Check sheet for the modelled part. Datum: model origin and axes. Units: mm. A direction names the side the tool comes from. Coordinates: 2 decimals unless noted, no trailing zeros. Loops run counter-clockwise (first coordinate to the right, second up) from the corner with the lowest first, then second, coordinate; pieces in that order, holes last. Notation, with made-up numbers: M 53,36.5 L 82,36.5 A10 cw 82,45.5 Z; hole C 73,18 d11. An arc over 180 degrees is marked long. Answer in a Markdown table with one row per item. Add a question column.
```python
from build123d import *

# Parameters (mm, degrees)
F0_R     = 12.5
F1_DEPTH = 14
F2_R     = 12.5
F2_R_2   = 11
F3_DEPTH = 5
F4_R     = 1
F5_DEPTH = 14.001
F6_R     = 1
F7_SIZE  = 1


with BuildPart() as f1:
    # F0 (on Top) → F1 (new body)
    with BuildSketch(Plane.XY):
        Circle(F0_R)
        Polygon((5.1, 2.9444863729), (5.1, -2.9444863729), (0, -5.8889727457), (-5.1, -2.9444863729), (-5.1, 2.9444863729), (0, 5.8889727457), align=None, mode=Mode.SUBTRACT)
    extrude(amount=F1_DEPTH)

    # F2 (on face) → F3 (cut)
    with BuildSketch(Plane.XY.offset(14)):
        Circle(F2_R)
        Circle(F2_R_2, mode=Mode.SUBTRACT)
    extrude(amount=-F3_DEPTH, mode=Mode.SUBTRACT)

    # F4 (on face) → F5 (cut, through all)
    with BuildSketch(Plane.XY.offset(14)):
        with Locations((0, 5.1)):
            Circle(F4_R)
        with Locations((-4.4167295593, 2.55)):
            Circle(F4_R)
        with Locations((-4.4167295593, -2.55)):
            Circle(F4_R)
        with Locations((0, -5.1)):
            Circle(F4_R)
        with Locations((4.4167295593, -2.55)):
            Circle(F4_R)
        with Locations((4.4167295593, 2.55)):
            Circle(F4_R)
    extrude(amount=-F5_DEPTH, mode=Mode.SUBTRACT)

    # F6
    f6_edges = [f1.edges().sort_by_distance(p)[0] for p in [
        (-5.1, 1.819835, 7),
        (-5.1, -1.819835, 7),
        (-4.126023, -3.506812, 7),
        (-0.973977, -5.326647, 7),
        (0.973977, -5.326647, 7),
        (4.126023, -3.506812, 7),
        (5.1, -1.819835, 7),
        (5.1, 1.819835, 7),
        (4.126023, 3.506812, 7),
        (0.973977, 5.326647, 7),
        (-0.973977, 5.326647, 7),
        (-4.126023, 3.506812, 7),
    ]]
    fillet(f6_edges, radius=F6_R)

    # F7
    f7_edges = [f1.edges().sort_by_distance(p)[0] for p in [
        (-11, 0, 14),
        (-12.5, 0, 0),
    ]]
    chamfer(f7_edges, length=F7_SIZE)

    # F8 (on Right) → F9 (revolve, cut)
    with BuildSketch(Plane.YZ):
        with BuildLine():
            Line((0, 3), (0, -15))
            ThreePointArc((0, -15), (9, -6), (0, 3))
        make_face()
        with BuildLine():
            Line((0, 29), (0, 11))
            ThreePointArc((0, 11), (9, 20), (0, 29))
        make_face()
    revolve(axis=Axis((0, 0, -6), (0, 0, 1)), mode=Mode.SUBTRACT)


solid = f1.part
```
Q1. Cross-section at C-C (z = 3.5). Record the cut outline in (x, y), plus the area to 3 significant figures.
Q2. Access from +Z, -Z, +X, -X, +Y, -Y to the whole of each face (thin tool, end or side, straight path). Record for faces 5 (the face through (7, -2, 14)), 6 (the face through (-5.1, 0, 7)).
Q3. Mould release check, pull along Y, two halves, no side actions. Record for faces 1 (the face through (5.1, 0, 7)), 2 (the face through (2.53, 4.43, 6.92)), 3 (the face through (-2.38, -10.74, 11.03)), 4 (the face through (5, -10, 9)): released by +Y, released by -Y, zero draft, split by the parting line, or undercut.
Q4. Go/stop test with flat-tipped pins: pin 1 (1.5 mm diameter, centred on y = -0.5, z = 6, fed in from +X); pin 2 (6 mm diameter, centred on x = 9, z = 3.5, fed in from -Y); pin 3 (2 mm diameter, centred on x = -7.5, z = 3.5, fed in from +Y). Record where each tip stops, or that it passes through.
Q5. Thickness scan on L1, parallel to X at y = 0.25, z = 4.75; L2, parallel to Y at x = 9.75, z = 10.75; L3, parallel to Y at x = 0, z = 13.5. Record the ranges inside material, lowest first.
Q6. Cross-section at B-B (y = 0). Record the cut outline in (x, z).
Q7. Cross-section at A-A (x = 0). Record the cut outline in (y, z), plus the area to 3 significant figures.
Answer key:
| question | item | result |
|---|---|---|
| 1 | outline | C 0,0 d25; hole M -5.26,-2.01 A1 ccw -4.37,-3.55 A1 cw -3.82,-3.68 L -1.28,-5.15 A1 cw -0.89,-5.56 A1 ccw 0.89,-5.56 A1 cw 1.28,-5.15 L 3.82,-3.68 A1 cw 4.37,-3.55 A1 ccw 5.26,-2.01 A1 cw 5.1,-1.47 L 5.1,1.47 A1 cw 5.26,2.01 A1 ccw 4.37,3.55 A1 cw 3.82,3.68 L 1.28,5.15 A1 cw 0.89,5.56 A1 ccw -0.89,5.56 A1 cw -1.28,5.15 L -3.82,3.68 A1 cw -4.37,3.55 A1 ccw -5.26,2.01 A1 cw -5.1,1.47 L -5.1,-1.47 A1 cw Z |
| 1 | area | 397 mm^2 |
| 2 | face 5 | +Z, +X, -X, +Y, -Y |
| 2 | face 6 | +Z, -Z |
| 3 | face 1 | undercut |
| 3 | face 2 | undercut |
| 3 | face 3 | split by the parting line |
| 3 | face 4 | zero draft |
| 4 | pin 1 | x = 12.5 |
| 4 | pin 2 | y = -10.97 |
| 4 | pin 3 | y = 10.68 |
| 5 | L1 | -12.5 to -5.1, 5.1 to 12.5 |
| 5 | L2 | -5.09 to 5.09 |
| 5 | L3 | -10.5 to -6.22, 6.22 to 10.5 |
| 6 | outline | M -12.5,1 L -11.5,0 L -6.71,0 A9 cw -5.1,1.42 L -5.1,12.58 A9 cw -6.71,14 L -10,14 L -11,13 L -11,9 L -12.5,9 Z; M 5.1,1.42 A9 cw 6.71,0 L 11.5,0 L 12.5,1 L 12.5,9 L 11,9 L 11,13 L 10,14 L 6.71,14 A9 cw 5.1,12.58 Z |
| 7 | outline | M -12.5,1 L -11.5,0 L -6.71,0 A9 cw -6.1,0.62 L -6.1,13.38 A9 cw -6.71,14 L -10,14 L -11,13 L -11,9 L -12.5,9 Z; M 6.1,0.62 A9 cw 6.71,0 L 11.5,0 L 12.5,1 L 12.5,9 L 11,9 L 11,13 L 10,14 L 6.71,14 A9 cw 6.1,13.38 Z |
| 7 | area | 161 mm^2 |
